Here's the drawing with two shaded views (mm, measured from the low corner). I have some questions. Give positions to 0.01 mm unless a question says otherwise; leave off trailing zeros. Write each loop counter-clockwise with the first axis right and the second up, starting at its lowest first coordinate (ties: lowest second). Pieces come first, ordered by that corner, then holes. Notation, with made-up numbers: (1, 23.5) -> (23, 23.5) arc R23 cw to (23, 32.5) -> close; hole circle Ø6 at (11.5, 69.5). An arc over 180 degrees is marked (long way). One line per question, with ' | ' between items.
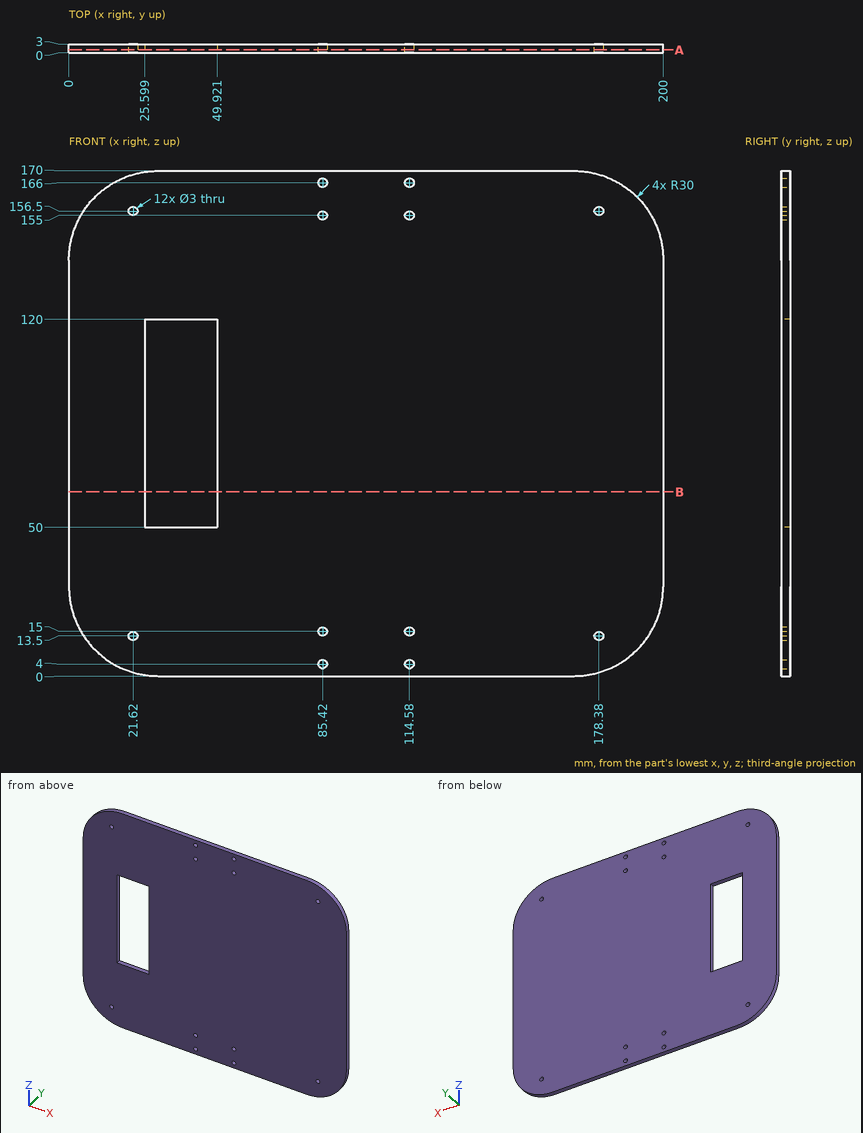
Q1. Will this pin go through, and if not, where does the flat tip stop? pin 1 (2.5 mm diameter, centred on x = 85.42, z = 15, fed in from -Y).
Answer below:
pin 1: passes through
Q2. Imagine slicing it at A-A on y = 1. Count the separate pieces of the cut face and the enclosed holes in it, and give its area (3 significant figures).
Answer below:
separate pieces: 1 | enclosed holes: 13 | area: 31,400 mm^2
Q3. If I drill on line 1 along Z through (x, y) = (114.58, 1.45); line 2 along Z through (x, y) = (32, 1.6); line 3 along X through (y, z) = (0.75, 4) (1 decimal), over which ranges is the centre line in solid material (lowest first)?
Answer below:
line 1: z = 0 to 2.5, 5.5 to 13.5, 16.5 to 153.5, 156.5 to 164.5, 167.5 to 170 | line 2: z = 0 to 50, 120 to 170 | line 3: x = 15 to 83.9, 86.9 to 113.1, 116.1 to 185
Q4. Imagine slicing it at B-B on z = 62. Please give me the cut outline in (x, y).
Answer below:
outline: (0, 0) -> (25.6, 0) -> (25.6, 3) -> (0, 3) -> close; (49.92, 0) -> (200, 0) -> (200, 3) -> (49.92, 3) -> close
